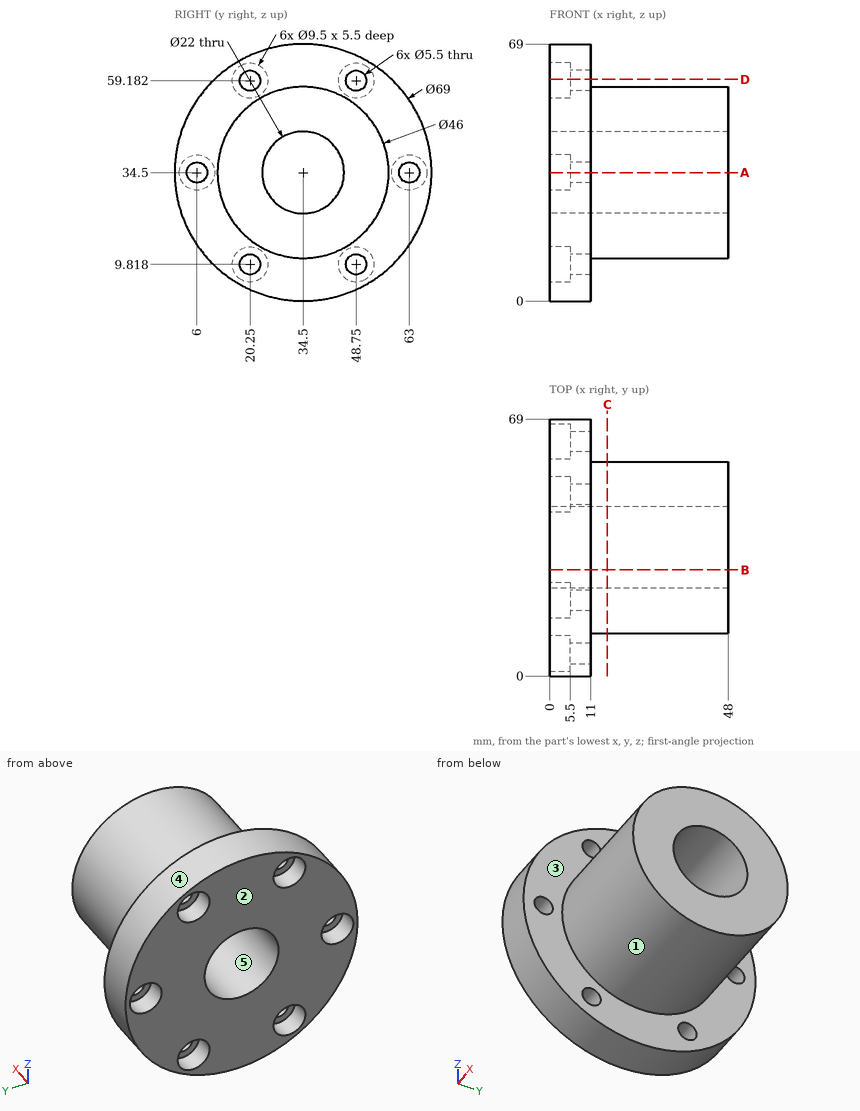
Source: three-view drawing plus pictorial views. Frame: mm from the lowest corner of the part. A direction names the side the tool comes from. Round coordinates to 2 decimals unless told otherwise and drop trailing zeros. Order: outer loops, then holes, each group sorted by start corner. A loop starts at its lowest first (then second) coordinate and runs counter-clockwise, first axis right, second up. Notation, with made-up numbers: (81.5, 73.5) -> (116.5, 73.5) arc R25 ccw to (116.5, 85.5) -> close; hole circle Ø11 at (-4.5, -16). An arc over 180 degrees is marked (long way). Use CSV: the item, a comma, the result in double quotes. Start each with the question number.
1) Draft query along Z for the marked faces 3, 4 and 5. Return one class per face: +Z half, -Z half, draft (parallel to the pull), parting line (faces both ways), or undercut.
2) Section C-C (x = 15.5). Return the cut outline in (y, z).
3) First-contact query: pin 1 Ø10 at (x, z) = (35, 21) entering from -Y; pin 2 Ø7.5 at (y, z) = (49, 59) entering from -X; pin 3 Ø3 at (y, z) = (26, 37.5) entering from +X; pin 4 Ø1 at (x, y) = (19.5, 56) entering from +Z. Flat tips, straight axial feed; report the tip coordinate or a pass-through.
4) Section D-D (z = 59.5). Return the cut outline in (x, y) (1 decimal), and give its area (3 significant figures).
5) Material intervals for line 1 along Z through (x, y) = (3.5, 17.5) (1 decimal); line 2 along Z through (x, y) = (9.15, 20.25); line 3 along X through (y, z) = (59, 23), sorted ascending. Write a range as from..to.
6) Section A-A (z = 34.5). Return the cut outline in (x, y), and give its area (3 significant figures).
7) Set-up query: the marked faces 1 and 2. Return all of +Z, -Z, +X, -X, +Y, -Y with unobstructed straight access to the full face (end or side cutting, diameter ignored); none if empty.
8) Section B-B (y = 28.5). Return the cut outline in (x, z).
Returned:
1,face 3,"draft"
1,face 4,"parting line"
1,face 5,"undercut"
2,outline,"circle Ø46 at (34.5, 34.5); hole circle Ø22 at (34.5, 34.5)"
3,pin 1,"stops at y = 13.13"
3,pin 2,"stops at x = 5.5"
3,pin 3,"passes through"
3,pin 4,"stops at z = 43.88"
4,outline,"(0, 10.7) -> (11, 10.7) -> (11, 17.5) -> (5.5, 17.5) -> (5.5, 15.5) -> (0, 15.5) -> close; (0, 25) -> (5.5, 25) -> (5.5, 23) -> (11, 23) -> (11, 46) -> (5.5, 46) -> (5.5, 44) -> (0, 44) -> close; (0, 53.5) -> (5.5, 53.5) -> (5.5, 51.5) -> (11, 51.5) -> (11, 58.3) -> (0, 58.3) -> close"
4,area,"359 mm²"
5,line 1,"z = 4.5..5.9, 13.7..55.3, 63.1..64.5"
5,line 2,"z = 3.08..7.07, 12.57..56.43, 61.93..65.92"
5,line 3,"x = 0..11"
6,outline,"(0, 0) -> (11, 0) -> (11, 3.25) -> (5.5, 3.25) -> (5.5, 1.25) -> (0, 1.25) -> close; (0, 10.75) -> (5.5, 10.75) -> (5.5, 8.75) -> (11, 8.75) -> (11, 11.5) -> (48, 11.5) -> (48, 23.5) -> (0, 23.5) -> close; (0, 45.5) -> (48, 45.5) -> (48, 57.5) -> (11, 57.5) -> (11, 60.25) -> (5.5, 60.25) -> (5.5, 58.25) -> (0, 58.25) -> close; (0, 67.75) -> (5.5, 67.75) -> (5.5, 65.75) -> (11, 65.75) -> (11, 69) -> (0, 69) -> close"
6,area,"1,240 mm²"
7,face 1,"+X"
7,face 2,"+Z, -Z, -X, +Y, -Y"
8,outline,"(0, 0.53) -> (11, 0.53) -> (11, 12.3) -> (48, 12.3) -> (48, 25.28) -> (0, 25.28) -> close; (0, 43.72) -> (48, 43.72) -> (48, 56.7) -> (11, 56.7) -> (11, 68.47) -> (0, 68.47) -> close"
